Geometry: final body of the model. Coordinates: model frame, mm. Face numbers are marked on the shaded views. A direction names the side the tool comes from. Round coordinates to 2 decimals unless told otherwise and drop trailing zeros. Loops run counter-clockwise (first coordinate to the right, second up) from the corner with the lowest first, then second, coordinate; pieces in that order, holes last. Notation, with made-up numbers: (-27, 65.5) - (-7, 65.5) arc R28 cw to (-7, 83.5) - close; hole circle Ø11 at (3, -26.75). An arc over 180 degrees is marked (long way). Answer as CSV lines item,"result".
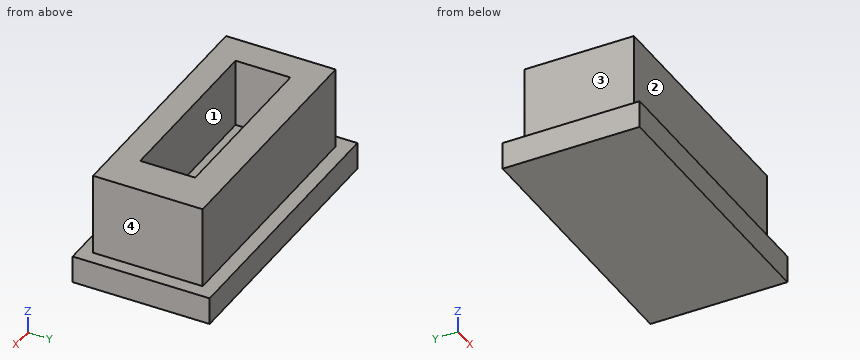
from build123d import *

# Parameters (mm, degrees)
F0_W     = 100
F0_H     = 50
F1_DEPTH = 10
F2_W     = 90
F2_H     = 40
F3_DEPTH = 5
F4_W     = 90
F4_H     = 40
F4_W_2   = 64.491807
F4_H_2   = 20.034401
F5_DEPTH = 25


with BuildPart() as f1:
    # F0 (on Top) → F1 (new body)
    with BuildSketch(Plane.XY):
        with Locations((-2.130391, -9.130959)):
            Rectangle(F0_W, F0_H)
    extrude(amount=F1_DEPTH)

    # F2 (on face) → F3 (join)
    with BuildSketch(Plane.XY.offset(10)):
        with Locations((-2.126822, -9.367195)):
            Rectangle(F2_W, F2_H)
    extrude(amount=F3_DEPTH)

    # F4 (on face) → F5 (join)
    with BuildSketch(Plane.XY.offset(15)):
        with Locations((-2.126822, -9.367195)):
            Rectangle(F4_W, F4_H)
        with Locations((-3.999688, -10.0172)):
            Rectangle(F4_W_2, F4_H_2, mode=Mode.SUBTRACT)
    extrude(amount=F5_DEPTH)


solid = f1.part
(1) Section D-D (y = -15.5). Output: boundary loops of the cut face in (x, z).
Findings below:
outline,"(-52.13, 0) - (47.87, 0) - (47.87, 10) - (42.87, 10) - (42.87, 40) - (28.25, 40) - (28.25, 15) - (-36.25, 15) - (-36.25, 40) - (-47.13, 40) - (-47.13, 10) - (-52.13, 10) - close"
(2) Pin query (flat end, axial travel): P1, Ø20, axis at x = -1.5, z = 31.5, coming from the +Y side; P2, Ø16, axis at y = -6.5, z = 23.5, coming from the +X side; P3, Ø10, axis at y = -13.5, z = 32, coming from the -X side. Return the tip coordinate at first contact, or that it passes through.
Findings below:
P1,"y = 10.63"
P2,"x = 42.87"
P3,"x = -47.13"
(3) Access query for the marked faces 1, 2, 3 and 4. Directions: +Z, -Z, +X, -X, +Y, -Y. A direction counts if a zero-diameter tool reaches every point of the face in a straight line with its end or side. Return the directions, or none.
Findings below:
face 1,"+Z"
face 2,"+Z, +X, -X, -Y"
face 3,"+Z, -X, +Y, -Y"
face 4,"+Z, +X, +Y, -Y"
(4) Section B-B (z = 35.5). Output: boundary loops of the cut face in (x, y).
Findings below:
outline,"(-47.13, -29.37) - (42.87, -29.37) - (42.87, 10.63) - (-47.13, 10.63) - close; hole (-36.25, -20.03) - (28.25, -20.03) - (28.25, 0) - (-36.25, 0) - close"
(5) Section A-A (x = -39.5). Output: boundary loops of the cut face in (y, z).
Findings below:
outline,"(-34.13, 0) - (15.87, 0) - (15.87, 10) - (10.63, 10) - (10.63, 40) - (-29.37, 40) - (-29.37, 10) - (-34.13, 10) - close"
(6) Material intervals for line 1 along X through (y, z) = (-14.5, 30); line 2 along Y through (x, z) = (26, 18); line 3 along X through (y, z) = (3, 15), sorted ascending.
Findings below:
line 1,"-47.13 to -36.25, 28.25 to 42.87"
line 2,"-29.37 to -20.03, 0 to 10.63"
line 3,"-47.13 to 42.87"
(7) Section C-C (y = 8). Output: boundary loops of the cut face in (x, z).
Findings below:
outline,"(-52.13, 0) - (47.87, 0) - (47.87, 10) - (42.87, 10) - (42.87, 40) - (-47.13, 40) - (-47.13, 10) - (-52.13, 10) - close"
